Job drawing, mm, ordinate dimensions from the low corner. One solid piece. Round coordinates to 2 decimals unless told otherwise and drop trailing zeros. Write each loop counter-clockwise with the first axis right and the second up, starting at its lowest first coordinate (ties: lowest second). Pieces come first, ordered by that corner, then holes.
1) Saw through at B-B on x = 9.75. Write the cut outline in (y, z), and give its area (3 significant figures).
2) Drill centre line: L1, parallel to Z at x = 23.5, y = 25.25. Where is it in solid material? Low to high.
3) Saw through at A-A on z = 24. Write the cut outline in (x, y), and give its area (3 significant figures).
4) Pull direction Y, two halves, no side cores. Call the marked faces 1, 2 and 3: +Y half, -Y half, draft (parallel to the pull), parting line (faces both ways), or undercut.
5) Flat gauge pins, fed straight in: pin 1 (8 mm diameter, centred on x = 27, y = 22, fed in from -Z); pin 2 (6 mm diameter, centred on x = 24.5, z = 15, fed in from -Y). Where does each tip first touch, or does it go through?
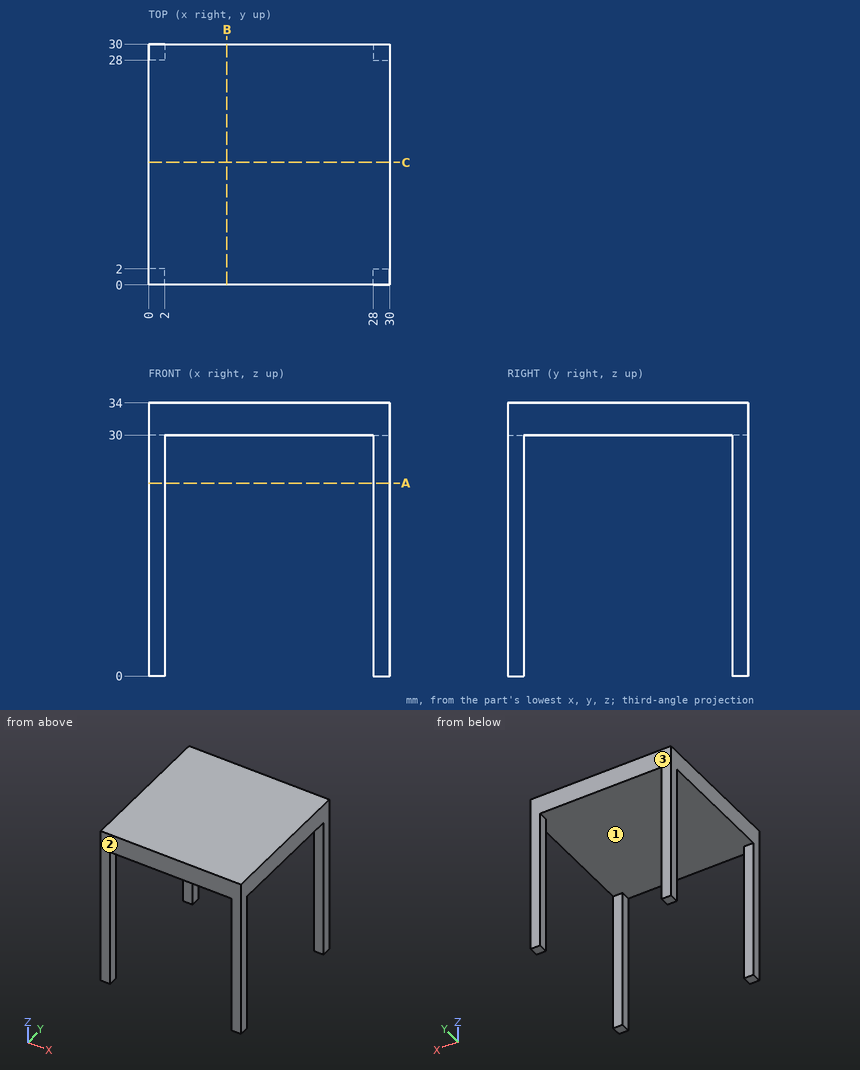
Completed:
1. outline: (0, 30) - (30, 30) - (30, 34) - (0, 34) - close
1. area: 120 mm2
2. L1: z = 30 to 34
3. outline: (0, 0) - (2, 0) - (2, 2) - (0, 2) - close; (0, 28) - (2, 28) - (2, 30) - (0, 30) - close; (28, 0) - (30, 0) - (30, 2) - (28, 2) - close; (28, 28) - (30, 28) - (30, 30) - (28, 30) - close
3. area: 16.0 mm2
4. face 1: undercut
4. face 2: -Y half
4. face 3: +Y half
5. pin 1: stops at z = 30
5. pin 2: passes through
